Here's how the part is built. I have some questions about the finished solid (model axes, mm). A direction names the side the tool comes from. Round coordinates to 2 decimals unless told otherwise and drop trailing zeros. Write each loop counter-clockwise with the first axis right and the second up, starting at its lowest first coordinate (ties: lowest second). Pieces come first, ordered by that corner, then holes. Notation, with made-up numbers: M 41,15 L 67,15 A18 ccw 67,34 Z; hole C -40,12.5 d2. An arc over 180 degrees is marked long. Write item = value, one per line. Start each with the question number.
(1) I want a section at D-D (y = -10.75). List the corners of the cut face in (x, z) for me, and give its area (3 significant figures).
(2) On a 3-axis mill with a long thin cutter (end or side, diameter ignored), from which of +Z, -Z, +X, -X, +Y, -Y can I reach the whole of each face in a straight line? I mean faces 5 (the flat face through (3, 1, 19.636)), 6 (the flat face through (3, -18, 19.636)), 7 (the flat face through (3, 5.537, 13)). Say none if no direction works.
(3) I want a section at C-C (z = 30.75). List the corners of the cut face in (x, y) for me.
(4) I want a section at B-B (x = 1.25). List the corners of the cut face in (y, z) for me (1 decimal).
(5) Will these pins go through, and if not, where does the flat tip stop? pin 1 Ø1.4 at (x, y) = (4.5, -17.5) entering from +Z; pin 2 Ø1.5 at (x, y) = (2, -3) entering from -Z; pin 3 Ø3 at (y, z) = (-8.75, 26.99) entering from -X; pin 4 Ø1.5 at (x, z) = (5, 25) entering from +Y.
(6) I need wall thicknesses on line 1 along Z through (x, y) = (3.5, -9); line 2 along Y through (x, z) = (2.5, 13); line 3 along Y through (x, z) = (2, 10.75). Which ranges of each line are inside material? Lowest first, please.
(7) If we mould it in two halves opening along Z, with no side actions, what happens to faces 1 (the cylindrical face through (3.131, -8.948, 14.286)), 2 (the cylindrical face through (3.13, -7.9, 21.98)), 3 (the flat face through (3, -4.305, 27)), 4 (the cylindrical face through (3.22, -13.96, 20.36))? For each: released by +Z, released by -Z, zero draft, split by the parting line, or undercut.
(8) I want a section at A-A (z = 13.25). List the corners of the cut face in (x, y) for me, and give its area (3 significant figures).
```python
from build123d import *

# Parameters (mm, degrees)
F0_R     = 1.5875
F1_DEPTH = 6.35
F2_R     = 1.27
F3_R     = 2.54


# Not quite as in the source:
# - a feature names something its author has since deleted; it is built from what else it names


with BuildPart() as f1:
    # F0 (on Right) → F1 (new body)
    with BuildSketch(Plane.YZ):
        with BuildLine():
            Line((-23.0375597417, 19.636290542), (-23.0375597417, 0))
            ThreePointArc((-23.0375597417, 0), (-8.7500597417, 14.2875), (5.5374402583, 0))
            Line((5.5374402583, 0), (5.5374402583, 19.636290542))
            Line((5.5374402583, 19.636290542), (-4.3050597417, 19.636290542))
            Line((-4.3050597417, 19.636290542), (-4.3050597417, 32.336290542))
            Line((-4.3050597417, 32.336290542), (-13.1950597417, 32.336290542))
            Line((-13.1950597417, 32.336290542), (-13.1950597417, 19.636290542))
            Line((-13.1950597417, 19.636290542), (-23.0375597417, 19.636290542))
        make_face()
        with Locations((-8.7500597417, 20.6375)):
            Circle(F0_R, mode=Mode.SUBTRACT)
        with Locations((-8.7500597417, 26.9875)):
            Circle(F0_R, mode=Mode.SUBTRACT)
    extrude(amount=F1_DEPTH)

    # F2
    f2_edges = [f1.edges().sort_by_distance(p)[0] for p in [
        (3.175, -23.03756, 0),
        (3.175, 5.53744, 0),
    ]]
    fillet(f2_edges, radius=F2_R)

    # F3
    f3_edges = [f1.edges().sort_by_distance(p)[0] for p in [
        (3.175, -23.03756, 19.636291),
        (3.175, 5.53744, 19.636291),
        (3.175, -4.30506, 19.636291),
        (3.175, -13.19506, 19.636291),
    ]]
    fillet(f3_edges, radius=F3_R)


solid = f1.part
```
Returned:
q1.outline = M 0,14.15 L 6.35,14.15 L 6.35,32.34 L 0,32.34 Z
q1.area = 116 mm²
q2.face_5 = +Z, +X, -X, +Y
q2.face_6 = +Z, +X, -X, -Y
q2.face_7 = +Z, -Z, +X, -X, +Y
q3.outline = M 0,-13.2 L 6.35,-13.2 L 6.35,-4.31 L 0,-4.31 Z
q4.outline = M -23,8.5 A1.3 ccw -20.7,7.8 A14.3 cw 3.2,7.8 A1.3 ccw 5.5,8.5 L 5.5,17.1 A2.5 ccw 3,19.6 L -1.8,19.6 A2.5 cw -4.3,22.2 L -4.3,32.3 L -13.2,32.3 L -13.2,22.2 A2.5 cw -15.7,19.6 L -20.5,19.6 A2.5 ccw -23,17.1 Z; hole C -8.8,20.6 d3.2; hole C -8.8,27 d3.2
q5.pin_1 = 19.64
q5.pin_2 = 12.72
q5.pin_3 = through
q5.pin_4 = -4.31
q6.line_1 = 14.29 to 19.07, 22.21 to 25.42, 28.56 to 32.34
q6.line_2 = -23.04 to -14.68, -2.82 to 5.54
q6.line_3 = -23.04 to -18.16, 0.66 to 5.54
q7.face_1 = released by -Z
q7.face_2 = undercut
q7.face_3 = zero draft
q7.face_4 = released by +Z
q8.outline = M 0,-23.04 L 6.35,-23.04 L 6.35,-14.1 L 0,-14.1 Z; M 0,-3.4 L 6.35,-3.4 L 6.35,5.54 L 0,5.54 Z
q8.area = 114 mm²
